Design review of the part built by this model. Coordinates are the model's own, in mm. A direction names the side the tool comes from. Coordinates: 2 decimals unless noted, no trailing zeros. Write each loop counter-clockwise with the first axis right and the second up, starting at its lowest first coordinate (ties: lowest second). Pieces come first, ordered by that corner, then holes. Notation, with made-up numbers: M 52,66 L 99,66 A4 cw 99,71 Z; hole C 88.5,31 d9. An arc over 180 degrees is marked long. Write item = value, one per line.
```python
from build123d import *

# Parameters (mm, degrees)
SKETCH1_W           = 60
SKETCH1_H           = 48.6
BOSS_EXTRUDE1_DEPTH = 3.8
SKETCH3_R           = 17.5
BOSS_EXTRUDE3_DEPTH = 3.8
CUT_EXTRUDE2_REACH  = 5.8
BOSS_EXTRUDE4_START = -1.3
SKETCH2_W           = 61.45
SKETCH2_H           = 51.45
BOSS_EXTRUDE4_DEPTH = 1


with BuildPart() as part:
    # Sketch1 → Boss-Extrude1 (new body)
    with BuildSketch(Plane.XY):
        with Locations((-0.864197531, -0.7)):
            Rectangle(SKETCH1_W, SKETCH1_H)
    extrude(amount=BOSS_EXTRUDE1_DEPTH)

    # Sketch3 → Boss-Extrude3 (add)
    with BuildSketch(Plane.XY.offset(3.8)):
        with Locations((29.001697978, 0)):
            Circle(SKETCH3_R)
    extrude(amount=-BOSS_EXTRUDE3_DEPTH)

    # Sketch4 → Cut-Extrude2 (cut, up to next)
    with BuildSketch(Plane.XY.offset(3.8), mode=Mode.PRIVATE) as cut_extrude2_sk1:
        with BuildLine():
            Line((29.135802469, 9.499486163), (29.135802469, -9.499486163))
            ThreePointArc((29.135802469, -9.499486163), (38.635288633, 0), (29.135802469, 9.499486163))
        make_face()
    cut_extrude2_tool1 = extrude(cut_extrude2_sk1.sketch, amount=-CUT_EXTRUDE2_REACH, mode=Mode.PRIVATE) & part.part
    add(cut_extrude2_tool1.solids().sort_by_distance((33.16751, 0, 3.8))[0], mode=Mode.SUBTRACT)

    # Sketch2 → Boss-Extrude4 (add)
    with BuildSketch(Plane.XY.offset(3.8).offset(BOSS_EXTRUDE4_START)):
        with Locations((-1.589197531, -0.725)):
            Rectangle(SKETCH2_W, SKETCH2_H)
    extrude(amount=-BOSS_EXTRUDE4_DEPTH)


solid = part.part
```
Q1. Consider section D-D, the plane y = 7. State the section outline as (x, z) points, and give its area (3 significant figures).
Check result:
outline = M -32.31,1.5 L -30.86,1.5 L -30.86,0 L 29.14,0 L 29.14,3.8 L -30.86,3.8 L -30.86,2.5 L -32.31,2.5 Z; M 35.56,0 L 45.04,0 L 45.04,3.8 L 35.56,3.8 Z
area = 265 mm²
Q2. For P1, Ø1.1, axis at y = 22.5, z = 2.5, coming from the +X side; P2, Ø1.2, axis at x = -13.5, z = 0.5, coming from the -Y side; P3, Ø1, axis at x = 3.5, z = 3.5, coming from the +Y side, all flat-tipped, find the tip position at first contact; note any pin that passes through.
Check result:
P1 = 29.14
P2 = -25
P3 = 23.6
Q3. Consider section B-B, the plane x = 37.5. State the section outline as (y, z) points, and give its area (3 significant figures).
Check result:
outline = M -15.3,0 L -4.5,0 L -4.5,3.8 L -15.3,3.8 Z; M 4.5,0 L 15.3,0 L 15.3,3.8 L 4.5,3.8 Z
area = 82.0 mm²
Q4. Wall thickness on line 1 (X direction, y = -22.5, z = 1.75); line 2 (X direction, y = 4, z = 2); line 3 (Y direction, x = -11, z = 3): over which ranges is each line inside the solid? List them lowest first.
Check result:
line_1 = -32.31 to 29.14
line_2 = -32.31 to 29.14, 37.75 to 46.04
line_3 = -25 to 23.6
Q5. Consider section C-C, the plane y = 18.5. State the section outline as (x, z) points.
Check result:
outline = M -32.31,1.5 L -30.86,1.5 L -30.86,0 L 29.14,0 L 29.14,3.8 L -30.86,3.8 L -30.86,2.5 L -32.31,2.5 Z
Q6. Consider section A-A, the plane y = 0. State the section outline as (x, z) points, and give its area (3 significant figures).
Check result:
outline = M -32.31,1.5 L -30.86,1.5 L -30.86,0 L 29.14,0 L 29.14,3.8 L -30.86,3.8 L -30.86,2.5 L -32.31,2.5 Z; M 38.64,0 L 46.5,0 L 46.5,3.8 L 38.64,3.8 Z
area = 259 mm²
Q7. The part is to be moulded in two halves that separate along Y. For faces 1 (the flat face through (-1, 23.6, 1)), 2 (the flat face through (-1, -25, 1)), 3 (the cylindrical face through (38.633, -0.209, 1.927)), say which applies: +Y half, -Y half, draft (parallel to the pull), parting line (faces both ways), or undercut.
Check result:
face_1 = +Y half
face_2 = -Y half
face_3 = undercut
Q8. Machinability: for faces 4 (the flat face through (-30.864, -1, 1)), 5 (the flat face through (29.136, 0, 2)), 6 (the flat face through (29.136, 20, 2)), 7 (the flat face through (29.136, -21, 2)), which of the approach directions +Z, -Z, +X, -X, +Y, -Y give a long, thin tool a straight path to every point of the face, cutting with its end or side? Answer none if there is none.
Check result:
face_4 = -Z, -X, +Y, -Y
face_5 = +Z, -Z
face_6 = +Z, -Z, +X, +Y
face_7 = +Z, -Z, +X, -Y
